CAD build for the part. Positions are in the model's coordinates, mm. A direction names the side the tool comes from. Give positions to 0.01 mm unless a question says otherwise; leave off trailing zeros. Write each loop counter-clockwise with the first axis right and the second up, starting at its lowest first coordinate (ties: lowest second). Pieces come first, ordered by that corner, then holes. Notation, with made-up numbers: (53.25, 79) - (84.25, 79) arc R13 cw to (84.25, 102) - close; hole circle Ø1 at (62.5, 43). An arc over 180 degrees is marked (long way). Answer as a JSON object with one key per item and string values.
from build123d import *

# Parameters (mm, degrees)
SKETCH1_R           = 1.6
SKETCH1_R_2         = 1.59
SKETCH1_R_3         = 1.75
SKETCH1_W           = 10.1
SKETCH1_H           = 3.1
SKETCH1_W_2         = 3.1
SKETCH1_H_2         = 10.1
BOSS_EXTRUDE1_DEPTH = 3
CUT_EXTRUDE1_REACH  = 162.106
SKETCH3_R           = 1.35
SKETCH3_R_2         = 1.6
FILLET1_R           = 3


with BuildPart() as part:
    # Sketch1 → Boss-Extrude1 (new body)
    with BuildSketch(Plane(origin=(0, 0, 0), x_dir=(1, 0, 0), z_dir=(0, 1, 0))):
        Polygon((-85, 100), (85, 100), (125, 76.905989232), (125, -76.905989232), (85, -100), (-85, -100), (-125, -76.905989232), (-125, 76.905989232), align=None)
        with Locations(Location((-50.5, -63, 0), (0, 0, 270))):
            Circle(SKETCH1_R, mode=Mode.SUBTRACT)
        with Locations(Location((82.856406461, 92, 0), (0, 0, 270))):
            Circle(SKETCH1_R, mode=Mode.SUBTRACT)
        with Locations(Location((117, 72.287187079, 0), (0, 0, 270))):
            Circle(SKETCH1_R, mode=Mode.SUBTRACT)
        with Locations(Location((117, -72.287187079, 0), (0, 0, 270))):
            Circle(SKETCH1_R, mode=Mode.SUBTRACT)
        with Locations(Location((82.856406461, -92, 0), (0, 0, 270))):
            Circle(SKETCH1_R, mode=Mode.SUBTRACT)
        with Locations(Location((-24.5, -63, 0), (0, 0, 270))):
            Circle(SKETCH1_R, mode=Mode.SUBTRACT)
        with Locations(Location((-24.5, 60, 0), (0, 0, 270))):
            Circle(SKETCH1_R, mode=Mode.SUBTRACT)
        with Locations(Location((-117, -72.287187079, 0), (0, 0, 270))):
            Circle(SKETCH1_R, mode=Mode.SUBTRACT)
        with Locations(Location((-50.5, -92, 0), (0, 0, 270))):
            Circle(SKETCH1_R, mode=Mode.SUBTRACT)
        with Locations(Location((-50.5, 60, 0), (0, 0, 270))):
            Circle(SKETCH1_R, mode=Mode.SUBTRACT)
        with Locations(Location((-117, 72.287187079, 0), (0, 0, 270))):
            Circle(SKETCH1_R, mode=Mode.SUBTRACT)
        with Locations(Location((-50.5, 92, 0), (0, 0, 270))):
            Circle(SKETCH1_R, mode=Mode.SUBTRACT)
        with Locations(Location((-82.856406461, -92, 0), (0, 0, 270))):
            Circle(SKETCH1_R, mode=Mode.SUBTRACT)
        with Locations(Location((-82.856406461, 92, 0), (0, 0, 270))):
            Circle(SKETCH1_R, mode=Mode.SUBTRACT)
        with Locations(Location((-55, 71.5, 0), (0, 0, 270))):
            Circle(SKETCH1_R_2, mode=Mode.SUBTRACT)
        with Locations(Location((-76, 71.5, 0), (0, 0, 270))):
            Circle(SKETCH1_R_2, mode=Mode.SUBTRACT)
        with Locations(Location((-55, 83.5, 0), (0, 0, 90))):
            Circle(SKETCH1_R_2, mode=Mode.SUBTRACT)
        with Locations(Location((-76, 83.5, 0), (0, 0, 90))):
            Circle(SKETCH1_R_2, mode=Mode.SUBTRACT)
        with Locations(Location((-55, -83.5, 0), (0, 0, 270))):
            Circle(SKETCH1_R_2, mode=Mode.SUBTRACT)
        with Locations(Location((-55, -71.5, 0), (0, 0, 90))):
            Circle(SKETCH1_R_2, mode=Mode.SUBTRACT)
        with Locations(Location((-76, -71.5, 0), (0, 0, 90))):
            Circle(SKETCH1_R_2, mode=Mode.SUBTRACT)
        with Locations(Location((-76, -83.5, 0), (0, 0, 270))):
            Circle(SKETCH1_R_2, mode=Mode.SUBTRACT)
        with Locations(Location((37.707416379, 78.475, 0), (0, 0, 270))):
            Circle(SKETCH1_R_3, mode=Mode.SUBTRACT)
        with Locations(Location((58.457416379, 78.475, 0), (0, 0, 270))):
            Circle(SKETCH1_R_3, mode=Mode.SUBTRACT)
        with Locations((-22.45, -93.45)):
            Rectangle(SKETCH1_W, SKETCH1_H, mode=Mode.SUBTRACT)
        with Locations((-118.45, 60)):
            Rectangle(SKETCH1_W_2, SKETCH1_H_2, mode=Mode.SUBTRACT)
        with Locations((-118.45, 20)):
            Rectangle(SKETCH1_W_2, SKETCH1_H_2, mode=Mode.SUBTRACT)
        with Locations((-118.45, -20)):
            Rectangle(SKETCH1_W_2, SKETCH1_H_2, mode=Mode.SUBTRACT)
        with Locations((-118.45, -60)):
            Rectangle(SKETCH1_W_2, SKETCH1_H_2, mode=Mode.SUBTRACT)
        with Locations((118.45, -60)):
            Rectangle(SKETCH1_W_2, SKETCH1_H_2, mode=Mode.SUBTRACT)
        with Locations((118.45, -20)):
            Rectangle(SKETCH1_W_2, SKETCH1_H_2, mode=Mode.SUBTRACT)
        with Locations((118.45, 20)):
            Rectangle(SKETCH1_W_2, SKETCH1_H_2, mode=Mode.SUBTRACT)
        with Locations((118.45, 60)):
            Rectangle(SKETCH1_W_2, SKETCH1_H_2, mode=Mode.SUBTRACT)
        with Locations((22.45, -93.45)):
            Rectangle(SKETCH1_W, SKETCH1_H, mode=Mode.SUBTRACT)
        with Locations((67.35, -93.45)):
            Rectangle(SKETCH1_W, SKETCH1_H, mode=Mode.SUBTRACT)
        with Locations((67.35, 93.45)):
            Rectangle(SKETCH1_W, SKETCH1_H, mode=Mode.SUBTRACT)
        with Locations((22.45, 93.45)):
            Rectangle(SKETCH1_W, SKETCH1_H, mode=Mode.SUBTRACT)
        with Locations((-22.45, 93.45)):
            Rectangle(SKETCH1_W, SKETCH1_H, mode=Mode.SUBTRACT)
    extrude(amount=BOSS_EXTRUDE1_DEPTH)

    # Sketch3 → Cut-Extrude1 (cut, up to next)
    with BuildSketch(Plane(origin=(0, 3, 0), x_dir=(1, 0, 0), z_dir=(0, 1, 0)), mode=Mode.PRIVATE) as cut_extrude1_sk1:
        with Locations(Location((-100, -46, 0), (0, 0, 270))):
            Circle(SKETCH3_R)
    cut_extrude1_tool1 = extrude(cut_extrude1_sk1.sketch, amount=-CUT_EXTRUDE1_REACH, mode=Mode.PRIVATE) & part.part
    # Sketch3 → Cut-Extrude1 (cut, up to next)
    with BuildSketch(Plane(origin=(0, 3, 0), x_dir=(1, 0, 0), z_dir=(0, 1, 0)), mode=Mode.PRIVATE) as cut_extrude1_sk2:
        with Locations(Location((-42, -46, 0), (0, 0, 270))):
            Circle(SKETCH3_R)
    cut_extrude1_tool2 = extrude(cut_extrude1_sk2.sketch, amount=-CUT_EXTRUDE1_REACH, mode=Mode.PRIVATE) & part.part
    # Sketch3 → Cut-Extrude1 (cut, up to next)
    with BuildSketch(Plane(origin=(0, 3, 0), x_dir=(1, 0, 0), z_dir=(0, 1, 0)), mode=Mode.PRIVATE) as cut_extrude1_sk3:
        with Locations(Location((-42, 40, 0), (0, 0, 270))):
            Circle(SKETCH3_R)
    cut_extrude1_tool3 = extrude(cut_extrude1_sk3.sketch, amount=-CUT_EXTRUDE1_REACH, mode=Mode.PRIVATE) & part.part
    # Sketch3 → Cut-Extrude1 (cut, up to next)
    with BuildSketch(Plane(origin=(0, 3, 0), x_dir=(1, 0, 0), z_dir=(0, 1, 0)), mode=Mode.PRIVATE) as cut_extrude1_sk4:
        with Locations(Location((-100, 40, 0), (0, 0, 270))):
            Circle(SKETCH3_R)
    cut_extrude1_tool4 = extrude(cut_extrude1_sk4.sketch, amount=-CUT_EXTRUDE1_REACH, mode=Mode.PRIVATE) & part.part
    # Sketch3 → Cut-Extrude1 (cut, up to next)
    with BuildSketch(Plane(origin=(0, 3, 0), x_dir=(1, 0, 0), z_dir=(0, 1, 0)), mode=Mode.PRIVATE) as cut_extrude1_sk5:
        with Locations(Location((18, 61, 0), (0, 0, 270))):
            Circle(SKETCH3_R_2)
    cut_extrude1_tool5 = extrude(cut_extrude1_sk5.sketch, amount=-CUT_EXTRUDE1_REACH, mode=Mode.PRIVATE) & part.part
    # Sketch3 → Cut-Extrude1 (cut, up to next)
    with BuildSketch(Plane(origin=(0, 3, 0), x_dir=(1, 0, 0), z_dir=(0, 1, 0)), mode=Mode.PRIVATE) as cut_extrude1_sk6:
        with Locations(Location((105, 61, 0), (0, 0, 270))):
            Circle(SKETCH3_R_2)
    cut_extrude1_tool6 = extrude(cut_extrude1_sk6.sketch, amount=-CUT_EXTRUDE1_REACH, mode=Mode.PRIVATE) & part.part
    # Sketch3 → Cut-Extrude1 (cut, up to next)
    with BuildSketch(Plane(origin=(0, 3, 0), x_dir=(1, 0, 0), z_dir=(0, 1, 0)), mode=Mode.PRIVATE) as cut_extrude1_sk7:
        with Locations(Location((105, -61, 0), (0, 0, 270))):
            Circle(SKETCH3_R_2)
    cut_extrude1_tool7 = extrude(cut_extrude1_sk7.sketch, amount=-CUT_EXTRUDE1_REACH, mode=Mode.PRIVATE) & part.part
    # Sketch3 → Cut-Extrude1 (cut, up to next)
    with BuildSketch(Plane(origin=(0, 3, 0), x_dir=(1, 0, 0), z_dir=(0, 1, 0)), mode=Mode.PRIVATE) as cut_extrude1_sk8:
        with Locations(Location((18, -61, 0), (0, 0, 270))):
            Circle(SKETCH3_R_2)
    cut_extrude1_tool8 = extrude(cut_extrude1_sk8.sketch, amount=-CUT_EXTRUDE1_REACH, mode=Mode.PRIVATE) & part.part
    # Sketch3 → Cut-Extrude1 (cut, up to next)
    with BuildSketch(Plane(origin=(0, 3, 0), x_dir=(1, 0, 0), z_dir=(0, 1, 0)), mode=Mode.PRIVATE) as cut_extrude1_sk9:
        with BuildLine():
            Line((28, 56), (95, 56))
            ThreePointArc((95, 56), (98.535533906, 54.535533906), (100, 51))
            Line((100, 51), (100, -51))
            ThreePointArc((100, -51), (98.535533906, -54.535533906), (95, -56))
            Line((95, -56), (28, -56))
            ThreePointArc((28, -56), (24.464466094, -54.535533906), (23, -51))
            Line((23, -51), (23, 51))
            ThreePointArc((23, 51), (24.464466094, 54.535533906), (28, 56))
        make_face()
    cut_extrude1_tool9 = extrude(cut_extrude1_sk9.sketch, amount=-CUT_EXTRUDE1_REACH, mode=Mode.PRIVATE) & part.part
    # Sketch3 → Cut-Extrude1 (cut, up to next)
    with BuildSketch(Plane(origin=(0, 3, 0), x_dir=(1, 0, 0), z_dir=(0, 1, 0)), mode=Mode.PRIVATE) as cut_extrude1_sk10:
        with BuildLine():
            Line((-20, -50), (0, -50))
            ThreePointArc((0, -50), (3.535533906, -48.535533906), (5, -45))
            Line((5, -45), (5, -25))
            ThreePointArc((5, -25), (3.535533906, -21.464466094), (0, -20))
            Line((0, -20), (-20, -20))
            ThreePointArc((-20, -20), (-23.535533906, -21.464466094), (-25, -25))
            Line((-25, -25), (-25, -45))
            ThreePointArc((-25, -45), (-23.535533906, -48.535533906), (-20, -50))
        make_face()
    cut_extrude1_tool10 = extrude(cut_extrude1_sk10.sketch, amount=-CUT_EXTRUDE1_REACH, mode=Mode.PRIVATE) & part.part
    add(cut_extrude1_tool1.solids().sort_by_distance((-100, 3, 46))[0], mode=Mode.SUBTRACT)
    add(cut_extrude1_tool2.solids().sort_by_distance((-42, 3, 46))[0], mode=Mode.SUBTRACT)
    add(cut_extrude1_tool3.solids().sort_by_distance((-42, 3, -40))[0], mode=Mode.SUBTRACT)
    add(cut_extrude1_tool4.solids().sort_by_distance((-100, 3, -40))[0], mode=Mode.SUBTRACT)
    add(cut_extrude1_tool5.solids().sort_by_distance((18, 3, -61))[0], mode=Mode.SUBTRACT)
    add(cut_extrude1_tool6.solids().sort_by_distance((105, 3, -61))[0], mode=Mode.SUBTRACT)
    add(cut_extrude1_tool7.solids().sort_by_distance((105, 3, 61))[0], mode=Mode.SUBTRACT)
    add(cut_extrude1_tool8.solids().sort_by_distance((18, 3, 61))[0], mode=Mode.SUBTRACT)
    add(cut_extrude1_tool9.solids().sort_by_distance((61.5, 3, 0))[0], mode=Mode.SUBTRACT)
    add(cut_extrude1_tool10.solids().sort_by_distance((-10, 3, 35))[0], mode=Mode.SUBTRACT)

    # Fillet1
    fillet1_edges = [part.edges().sort_by_distance(p)[0] for p in [
        (-85, 1.5, -100),
        (85, 1.5, -100),
        (125, 1.5, -76.905989232),
        (125, 1.5, 76.905989232),
        (85, 1.5, 100),
        (-85, 1.5, 100),
        (-125, 1.5, 76.905989232),
        (-125, 1.5, -76.905989232),
    ]]
    fillet(fillet1_edges, radius=FILLET1_R)


solid = part.part
(1) Pull direction X, two halves, no side cores. Call faces 1 (the face through (-104.863, 1.479, -88.532)), 2 (the face through (3, 2, 49)), 3 (the face through (25, 2, 55)), 4 (the face through (104.33, 1.48, -88.84)): pulls with the +X half, pulls with the -X half, needs draft (parallel to the pull), parting line crosses it, or undercut.
Answer key:
{"face 1": "pulls with the -X half", "face 2": "undercut", "face 3": "undercut", "face 4": "pulls with the +X half"}
(2) 3-axis set-ups, long thin cutter, end or side, ignore diameter. For faces 5 (the face through (2, 3, -1)), 6 (the face through (99, 2, 54)): which of +Z, -Z, +X, -X, +Y, -Y reach the whole face in a straight line?
Answer key:
{"face 5": "+Z, -Z, +X, -X, +Y", "face 6": "+Y, -Y"}
(3) Probe L1, parallel to X at y = 0.3, z = -25; L2, parallel to Z at x = 21.5, y = 1.95; L3, parallel to X at y = 0.6, z = 63. List the from-to ranges inside material, lowest first. Write a range as [from, to].
Answer key:
{"L1": "x = [-125, -120], [-116.9, 23], [100, 116.9], [120, 125]", "L2": "z = [-100, -95], [-91.9, 91.9], [95, 100]", "L3": "x = [-125, -120], [-116.9, -52.1], [-48.9, -26.1], [-22.9, 116.9], [120, 125]"}
(4) Saw through at A-A, the plane z = 28.5. Give the cut face in (x, y).
Answer key:
{"outline": "(-125, 0) - (-25, 0) - (-25, 3) - (-125, 3) - close; (5, 0) - (23, 0) - (23, 3) - (5, 3) - close; (100, 0) - (125, 0) - (125, 3) - (100, 3) - close"}
(5) Saw through at B-B, the plane z = -7. Give the cut face in (x, y).
Answer key:
{"outline": "(-125, 0) - (23, 0) - (23, 3) - (-125, 3) - close; (100, 0) - (125, 0) - (125, 3) - (100, 3) - close"}
(6) Flat gauge pins, fed straight in: P1, Ø3, axis at x = 37.71, z = -78.47, coming from the +Y side; P2, Ø4, axis at x = -33.5, z = 4.5, coming from the -Y side; P3, Ø0.9, axis at x = 118, y = 1, coming from the -Z side. Where does each tip first touch, or does it go through?
Answer key:
{"P1": "passes through", "P2": "stops at y = 0", "P3": "stops at z = -81.21"}
(7) Saw through at C-C, the plane y = 0.65. State how many separate pieces and enclosed holes the cut face has, and give its area (3 significant figures).
Answer key:
{"separate pieces": "1", "enclosed holes": "48", "area": "38,000 mm²"}
